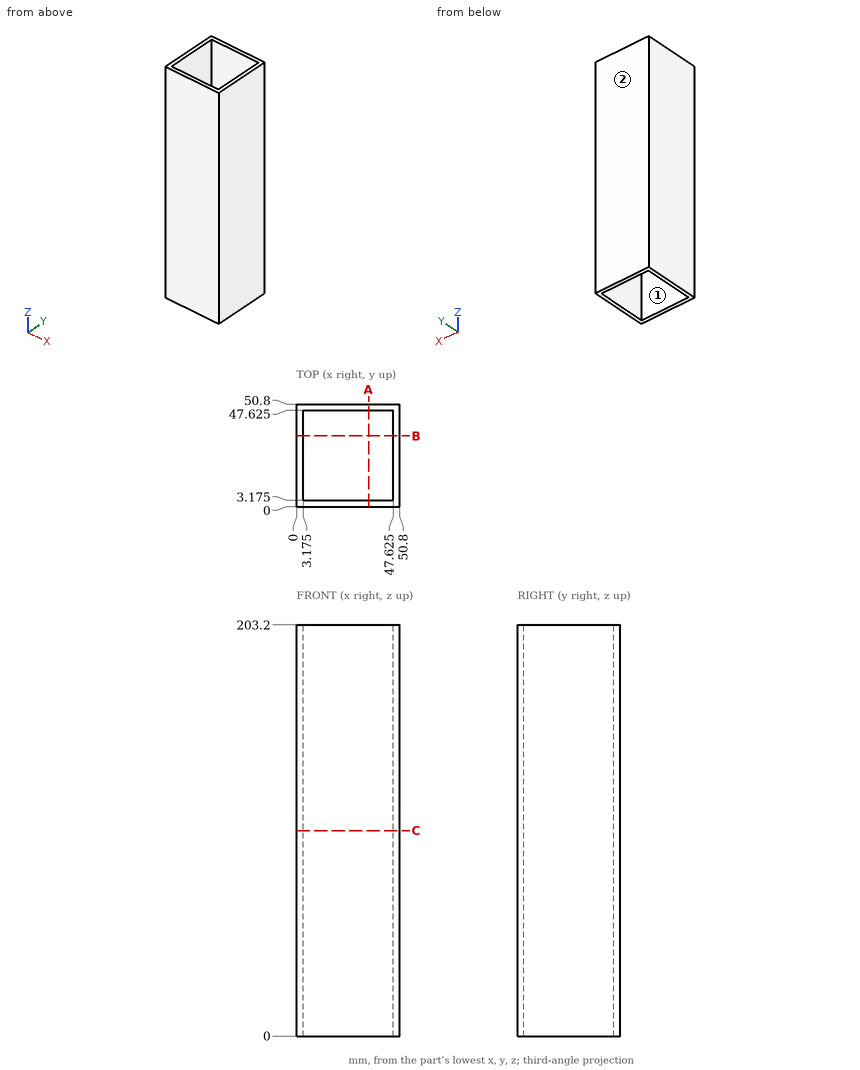
Geometry check sheet. Reference: drawing and pictorial views, mm from the part's lowest x, y, z. A direction names the side the tool comes from. Give positions to 0.01 mm unless a question says otherwise; leave off trailing zeros. Loops run counter-clockwise (first coordinate to the right, second up) from the corner with the lowest first, then second, coordinate; pieces in that order, holes last. Notation, with made-up numbers: (9, 10.5) - (25, 10.5) arc R27 cw to (25, 49.5) - close; hole circle Ø5 at (57, 83.5). An arc over 180 degrees is marked (long way). One line per question, with ' | ' between items. Start each with the question number.
1. Material ranges on line 1 along X through (y, z) = (27, 28) (3 decimals), recorded low to high. Write a range as [from, to].
2. Set-up check for the marked faces 1 and 2: record each of +Z, -Z, +X, -X, +Y, -Y from which the full face is reachable in a straight line by a thin tool's end or side.
3. Cross-section at A-A, the plane x = 35.5. Enter the section's corners in (y, z) (3 decimals).
4. Cross-section at C-C, the plane z = 101.5. Enter the section's corners in (x, y) (3 decimals).
5. Gauge pin test, flat end, axial feed: pin 1 Ø4 at (x, y) = (8.5, 44) entering from +Z. Record the tip position at first contact, or that the pin passes through.
Check result:
1) line 1: x = [0, 3.175], [47.625, 50.8]
2) face 1: +Z, -Z | face 2: +Z, -Z, +X, -X, +Y
3) outline: (0, 0) - (3.175, 0) - (3.175, 203.2) - (0, 203.2) - close; (47.625, 0) - (50.8, 0) - (50.8, 203.2) - (47.625, 203.2) - close
4) outline: (0, 0) - (50.8, 0) - (50.8, 50.8) - (0, 50.8) - close; hole (3.175, 3.175) - (47.625, 3.175) - (47.625, 47.625) - (3.175, 47.625) - close
5) pin 1: passes through
